Can you work these out from the model? Positions are in its coordinate system, mm. Face numbers are marked on the shaded views. A direction names the side the tool comes from. Give positions to 0.01 mm unless a question says otherwise; leave off trailing zeros. Order: outer loops, then holes, each group sorted by start corner. A loop starts at its lowest first (then second) coordinate and runs counter-clockwise, first axis right, second up. Notation, with made-up numbers: M 9.5,6.25 L 24.5,6.25 A27 ccw 24.5,42.25 Z; hole C 77,37.5 d7. An arc over 180 degrees is marked long. Use one line per item in the form item = value. Start each with the question number.
1. I want a section at B-B, the plane y = 5.5. List the corners of the cut face in (x, z) for me (3 decimals).
2. We'd pull the mould along X, two halves only. Please class the marked faces 3, 4 and 5: +X half, -X half, draft (parallel to the pull), parting line (faces both ways), or undercut.
3. I want a section at C-C, the plane z = -7. List the corners of the cut face in (x, y) for me, and give its area (3 significant figures).
4. I want a section at D-D, the plane x = -6.5. List the corners of the cut face in (y, z) for me.
5. Will these pins go through, and if not, where does the flat tip stop? P1, Ø3, axis at y = 5, z = 2, coming from the +X side; P2, Ø1.5, axis at x = 9.5, y = 9, coming from the -Z side; P3, Ø2, axis at y = 3.5, z = -3, coming from the +X side.
6. For the marked faces 1 and 2, which set-ups out of +Z, -Z, +X, -X, +Y, -Y let a thin tool reach every point of the face, with its end or its side?
7. I need wall thicknesses on L1, parallel to X at y = 1, z = -3.5; L2, parallel to X at y = 8.75, z = -5.5; L3, parallel to Z at x = 15.5, y = 11. Which ranges of each line are inside material? Lowest first, please.
8. I want a section at A-A, the plane z = -3. List the corners of the cut face in (x, y) for me, and give its area (3 significant figures).
```python
from build123d import *

# Parameters (mm, degrees)
BOSS_EXTRUDE1_DEPTH = 12.7


with BuildPart() as part:
    # Sketch1 → Boss-Extrude1 (new body)
    with BuildSketch(Plane(origin=(0, 0, 0), x_dir=(1, 0, 0), z_dir=(0, 1, 0))):
        with BuildLine():
            Line((0, 0), (16.497783942, 9.525))
            Line((16.497783942, 9.525), (18.402783942, 6.225443212))
            Line((18.402783942, 6.225443212), (10.153891971, 1.462943212))
            ThreePointArc((10.153891971, 1.462943212), (8.176843255, -3.633682641), (3.175, -5.839556788))
            Line((3.175, -5.839556788), (-3.175, -5.839556788))
            ThreePointArc((-3.175, -5.839556788), (-8.176843255, -3.633682641), (-10.153891971, 1.462943212))
            Line((-10.153891971, 1.462943212), (-18.402783942, 6.225443212))
            Line((-18.402783942, 6.225443212), (-16.497783942, 9.525))
            Line((-16.497783942, 9.525), (0, 0))
        make_face()
    extrude(amount=BOSS_EXTRUDE1_DEPTH)


solid = part.part
```
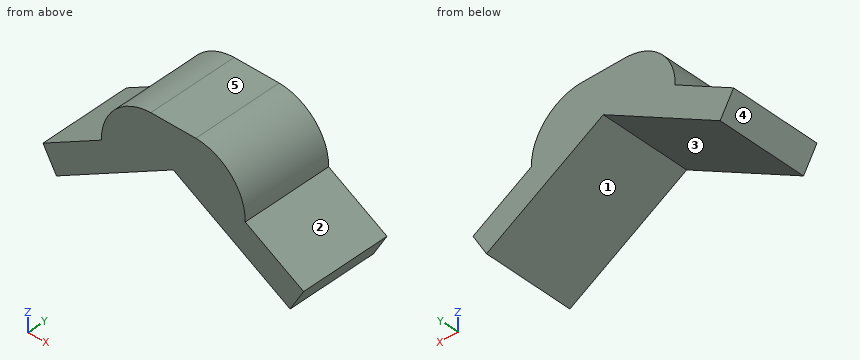
Check result:
q1.outline = M -18.403,-6.225 L -16.498,-9.525 L 0,0 L 16.498,-9.525 L 18.403,-6.225 L 10.154,-1.463 A7.143 ccw 3.175,5.84 L -3.175,5.84 A7.143 ccw -10.154,-1.463 Z
q2.face_3 = undercut
q2.face_4 = -X half
q2.face_5 = draft
q3.outline = M -17.96,0 L -12.12,0 L -12.12,12.7 L -17.96,12.7 Z; M 12.12,0 L 17.96,0 L 17.96,12.7 L 12.12,12.7 Z
q3.area = 148 mm2
q4.outline = M 0,-3.75 L 12.7,-3.75 L 12.7,4.93 L 0,4.93 Z
q5.P1 = 9.92
q5.P2 = -5.92
q5.P3 = 14.55
q6.face_1 = -Z, +Y, -Y
q6.face_2 = +Z, +X, +Y, -Y
q7.L1 = -13.68 to -6.06, 6.06 to 13.68
q7.L2 = -17.15 to -9.53, 9.53 to 17.15
q7.L3 = -8.95 to -4.55
q8.outline = M -12.82,0 L -5.2,0 L -5.2,12.7 L -12.82,12.7 Z; M 5.2,0 L 12.82,0 L 12.82,12.7 L 5.2,12.7 Z
q8.area = 194 mm2
